from build123d import *

# Parameters (mm, degrees)
BOSS_EXTRUDE1_DEPTH = 3.2004
SKETCH2_R           = 3.429
CUT_EXTRUDE1_DEPTH  = 3.2004
BOSS_EXTRUDE2_START = -3.2004
BOSS_EXTRUDE2_DEPTH = 3.2004
SKETCH4_R           = 6.35
CUT_EXTRUDE2_DEPTH  = 3.2004
FILLET1_R           = 12.7


with BuildPart() as part:
    # Sketch1 → Boss-Extrude1 (new body)
    with BuildSketch(Plane.XY):
        with BuildLine():
            ThreePointArc((-8.097097761, 15.832735205), (68.150612211, 34.198640293), (144.398322183, 15.832735205))
            ThreePointArc((144.398322183, 15.832735205), (152.133959628, -8.097097761), (128.204126662, -15.832735205))
            ThreePointArc((128.204126662, -15.832735205), (68.150612211, -1.367551307), (8.097097761, -15.832735205))
            ThreePointArc((8.097097761, -15.832735205), (-15.832735205, -8.097097761), (-8.097097761, 15.832735205))
        make_face()
    extrude(amount=BOSS_EXTRUDE1_DEPTH)

    # Sketch2 → Cut-Extrude1 (cut)
    with BuildSketch(Plane.XY.offset(3.2004)):
        with Locations((6.261836343, 3.437760818)):
            Circle(SKETCH2_R)
    extrude(amount=-CUT_EXTRUDE1_DEPTH, mode=Mode.SUBTRACT)

    # Sketch3 → Boss-Extrude2 (add)
    with BuildSketch(Plane.XY.offset(3.2004).offset(BOSS_EXTRUDE2_START)):
        with BuildLine():
            ThreePointArc((118.558560015, 1.198480685), (137.499705108, 17.742664408), (154.04388883, -1.198480685))
            ThreePointArc((154.04388883, -1.198480685), (151.248704167, -22.371604894), (145.781416871, -43.0167742))
            ThreePointArc((145.781416871, -43.0167742), (123.276823543, -54.242649292), (112.05094845, -31.738055964))
            ThreePointArc((112.05094845, -31.738055964), (116.357042584, -15.477699112), (118.558560015, 1.198480685))
        make_face()
    extrude(amount=BOSS_EXTRUDE2_DEPTH)

    # Sketch4 → Cut-Extrude2 (cut)
    with BuildSketch(Plane.XY.offset(3.2004)):
        with Locations((130.361522506, -37.860704571)):
            Circle(SKETCH4_R)
    extrude(amount=-CUT_EXTRUDE2_DEPTH, mode=Mode.SUBTRACT)

    # Fillet1
    fillet1_edges = [part.edges().sort_by_distance(p)[0] for p in [
        (117.190242121, -10.823434725, 1.6002),
    ]]
    fillet(fillet1_edges, radius=FILLET1_R)


solid = part.part
Can you work these out from the model? Positions are in its coordinate system, mm. Give positions to 0.01 mm unless a question says otherwise; leave off trailing zeros. Loops run counter-clockwise (first coordinate to the right, second up) from the corner with the lowest first, then second, coordinate; pieces in that order, holes last. Notation, with made-up numbers: M -16,76 L -7,76 A19 ccw -7,93 Z; hole C 44.5,76.25 d8. An arc over 180 degrees is marked long. One line per item, written item: value.
1) Imagine slicing it at D-D on x = 33. Write out the boundary of the cut face in (y, z).
Geometry check:
outline: M -6.14,0 L 30.47,0 L 30.47,3.2 L -6.14,3.2 Z
2) Imagine slicing it at B-B on z = 0.8. Count the separate pieces of the cut face and the enclosed holes in it, and give its area (3 significant figures).
Geometry check:
separate pieces: 1
enclosed holes: 2
area: 7,220 mm²
3) Imagine slicing it at C-C on y = -5. Write out the boundary of the cut face in (x, z), and give its area (3 significant figures).
Geometry check:
outline: M -17.07,0 L 37.41,0 L 37.41,3.2 L -17.07,3.2 Z; M 98.89,0 L 153.74,0 L 153.74,3.2 L 98.89,3.2 Z
area: 350 mm²
4) Please list where these lines run through material, in increasing order: line 1 (Y direction, x = 6.5, z = 1.05); line 2 (Y direction, x = 132, z = 0.65); line 3 (X direction, y = -16, z = 2.05).
Geometry check:
line 1: y = -16.55 to 0.02, 6.86 to 22.44
line 2: y = -54.89 to -44, -31.73 to 21.55
line 3: x = -7.76 to 7.76, 114.83 to 152.38
5) Imagine slicing it at A-A on y = -35. Write out the boundary of the cut face in (x, z).
Geometry check:
outline: M 111.29,0 L 124.69,0 L 124.69,3.2 L 111.29,3.2 Z; M 136.03,0 L 148.24,0 L 148.24,3.2 L 136.03,3.2 Z
6) I'm going to push flat-ended pins straight in: pin 1 (1.5 mm diameter, centred on x = 34.5, z = 0.5, fed in from -Y); pin 2 (1 mm diameter, centred on x = 134, z = 0.5, fed in from -Y). Where does each tip first touch, or does it pass through?
Geometry check:
pin 1: stops at y = -5.93
pin 2: stops at y = -54.56
7) Thinking about a two-plate mould opening in X: for faces 1 (the face through (113.512, -27.084, 1.578)), 2 (the face through (123.649, -54.363, 1.578)), 3 (the face through (133.292, -43.494, 1.623)), which applies, +X half, -X half, draft (parallel to the pull), parting line (faces both ways), or undercut?
Geometry check:
face 1: -X half
face 2: parting line
face 3: undercut
